Autodesk Inventor part; units mm, degrees
ref_plane "YZ Plane" through (0, 0, 0) normal (1, 0, 0) x (0, 1, 0)
ref_plane "XZ Plane" through (0, 0, 0) normal (0, 1, 0) x (-1, 0, 0)
ref_plane "XY Plane" through (0, 0, 0) normal (0, 0, 1) x (1, 0, 0)
sketch "Sketch1" plane through (0, 0, 0) normal (1, 0, 0) x (0, 1, 0)
  circle A0 centre (0, 0) radius 1.75
  circle A1 centre (0, 0) radius 3.5
  dimension "d0" = 3.5
  dimension "d1" = 7
extrude "Extrusion1" add sketch "Sketch1" along normal blind 3.5
sketch "Sketch2" plane through (3.5, 0, 0) normal (1, 0, 0) x (0, 0, -1)
  circle A0 centre (0, 0) radius 3.5 construction
  line L0 (0, 3.5) -> (0, 2.5) construction
  line L1 (0, 2.5) -> (1.5, 2.5) construction
  line L2 (1.5, 2.5) -> (-1.5, 2.5) construction
  line L3 (0, 3.5) -> (0, 6.5) construction
  line L4 (0, 6.5) -> (-1.5, 2.5)
  line L5 (0, 6.5) -> (2, 6.5)
  line L6 (2, 6.5) -> (0.5, 2.5)
  line L7 (-1.5, 2.5) -> (0.5, 2.5)
  dimension "d4" = 1
  dimension "d5" = 1.5
  dimension "d6" = 3
  dimension "d7" = 3
  dimension "d8" = 2
extrude "Extrusion2" add sketch "Sketch2" against normal blind 3.5
pattern_circular "Circular Pattern1" count 6 over 360 about axis through (0, 0, 0) along (1, 0, 0) of "Extrusion2"
properties part number "mtv_gear6v2_1-16"
Can you work these out from the model? Positions are in its coordinate system, mm. A direction names the side the tool comes from. Coordinates: 2 decimals unless noted, no trailing zeros. Order: outer loops, then holes, each group sorted by start corner. A loop starts at its lowest first (then second) coordinate and runs counter-clockwise, first axis right, second up. Notation, with made-up numbers: (70.25, 73.25) - (89.25, 73.25) arc R21 cw to (89.25, 101.25) - close; hole circle Ø8 at (65, 15.25). An arc over 180 degrees is marked (long way). Answer in a Markdown table with one row per item.
1. If I drill on line 1 along Z through (x, y) = (2.25, 0); line 2 along Y through (x, z) = (3.05, 4.25); line 3 along Y through (x, z) = (2.5, -3.75), over which ranges is the centre line in solid material (lowest first)?
Reply:
| item | result |
|---|---|
| line 1 | z = -3.5 to -1.75, 1.75 to 3.5 |
| line 2 | y = -3.02 to -1.12, 1.57 to 4.52 |
| line 3 | y = -3.91 to -0.97, 1.04 to 2.94 |
2. Suppose I cut it at C-C (z = 1). Please give me the cut outline in (x, y).
Reply:
| item | result |
|---|---|
| outline | (0, -6.5) - (3.5, -6.5) - (3.5, -3.83) - (0, -3.83) - close; (0, -3.35) - (3.5, -3.35) - (3.5, -1.44) - (0, -1.44) - close; (0, 1.44) - (3.5, 1.44) - (3.5, 3.83) - (0, 3.83) - close |
3. Suppose I cut it at B-B (y = 0). Please give me the cut outline in (x, z).
Reply:
| item | result |
|---|---|
| outline | (0, -3.5) - (3.5, -3.5) - (3.5, -1.75) - (0, -1.75) - close; (0, 1.75) - (3.5, 1.75) - (3.5, 3.5) - (0, 3.5) - close |
4. If we mould it in two halves opening along Z, with no side actions, what happens to faces 1 (the flat face through (1.77, 3.72, 3.59)), 2 (the flat face through (1.77, -1.25, 5.02)), 3 (the flat face through (1.77, 2.4, -6.12))? For each: pulls with the +Z half, pulls with the -Z half, needs draft (parallel to the pull), parting line crosses it, or undercut.
Reply:
| item | result |
|---|---|
| face 1 | undercut |
| face 2 | pulls with the +Z half |
| face 3 | pulls with the -Z half |
5. For pin 1 (3 mm diameter, centred on y = 0, z = 0, fed in from -X), with a flat end and sliding along its axis, tell me the tip position at first contact or that it passes through.
Reply:
| item | result |
|---|---|
| pin 1 | passes through |
6. Suppose I cut it at D-D (z = 3). Please give me the cut outline in (x, y).
Reply:
| item | result |
|---|---|
| outline | (0, -2.81) - (3.5, -2.81) - (3.5, 3) - (0, 3) - close |
7. Suppose I cut it at A-A (x = 1.25). Please give me the cut outline in (y, z), and give its area (3 significant figures).
Reply:
| item | result |
|---|---|
| outline | (-6.5, 0) - (-3.29, -1.21) arc R3.5 ccw to (-2.42, -2.52) - (-4.98, -4.63) - (-3.25, -5.63) - (-0.6, -3.45) arc R3.5 ccw to (0.97, -3.36) - (1.52, -6.63) - (3.25, -5.63) - (2.69, -2.24) arc R3.5 ccw to (3.4, -0.84) - (6.5, -2) - (6.5, 0) - (3.29, 1.21) arc R3.5 ccw to (2.42, 2.52) - (4.98, 4.63) - (3.25, 5.63) - (0.6, 3.45) arc R3.5 ccw to (-0.97, 3.36) - (-1.52, 6.63) - (-3.25, 5.63) - (-2.69, 2.24) arc R3.5 ccw to (-3.4, 0.84) - (-6.5, 2) - close; hole circle Ø3.5 at (0, 0) |
| area | 65.5 mm^2 |
8. For faces 4 (the flat face through (1.774, -2.972, 3.96)), 5 (the flat face through (1.77, -1.94, -4.55)), 6 (the flat face through (1.774, -4.971, 1.427)), which set-ups out of +Z, -Z, +X, -X, +Y, -Y let a thin tool reach every point of the face, with its end or its side?
Reply:
| item | result |
|---|---|
| face 4 | +X, -X, -Y |
| face 5 | -Z, +X, -X |
| face 6 | +Z, +X, -X |
